```python
from build123d import *

# Parameters (mm, degrees)
SKETCH1_RX               = 240
SKETCH1_RY               = 110
BOSS_EXTRUDE1_DEPTH      = 200
SKETCH12_R               = 9
CUT_EXTRUDE8_DEPTH       = 332.209903234
CUT_EXTRUDE10_DEPTH      = 332.209903234
CUT_EXTRUDE10_DEPTH_BACK = 332.209903234
SKETCH15_W               = 200
SKETCH15_H               = 15


with BuildPart() as part:
    # Sketch1 → Boss-Extrude1 (new body)
    with BuildSketch(Plane.XY):
        with Locations((0, 0)):
            Ellipse(SKETCH1_RX, SKETCH1_RY)
    extrude(amount=-BOSS_EXTRUDE1_DEPTH)

    # Sketch12 → Cut-Extrude8 (cut, through all)
    with BuildSketch(Plane.XY):
        with Locations((175, -30)):
            Circle(SKETCH12_R)
        with Locations(Location((-175, -30, 0), (0, 0, 180))):
            Circle(SKETCH12_R)
    extrude(amount=-CUT_EXTRUDE8_DEPTH, mode=Mode.SUBTRACT)

    # Sketch15 → Cut-Extrude10 (cut, two sides: drawn at the far end of the back side and taken through both)
    with BuildSketch(Plane(origin=(0, 0, 0), x_dir=(0, 0, -1), z_dir=(1, 0, 0)).offset(-CUT_EXTRUDE10_DEPTH_BACK)):
        Polygon((0, 110), (0, 95), (200, -5), (200, 110), align=None)
        with Locations((100, -102.5)):
            Rectangle(SKETCH15_W, SKETCH15_H)
    extrude(amount=CUT_EXTRUDE10_DEPTH + CUT_EXTRUDE10_DEPTH_BACK, mode=Mode.SUBTRACT)


solid = part.part
```
Check sheet for the modelled part. Datum: model origin and axes. Units: mm. Coordinates: 2 decimals unless noted, no trailing zeros. Write each loop counter-clockwise with the first axis right and the second up, starting at its lowest first coordinate (ties: lowest second). Pieces come first, ordered by that corner, then holes. Notation, with made-up numbers: M -20.5,66 L 11.5,66 A14 cw 11.5,76 Z; hole C -37,20.5 d11. An arc over 180 degrees is marked long. Write item = value, one per line. Start each with the question number.
1. Go/stop test with flat-tipped pins: pin 1 (5 mm diameter, centred on x = 161.5, z = -102.5, fed in from -Y); pin 2 (8 mm diameter, centred on x = -10, z = -89.5, fed in from +Y); pin 3 (10 mm diameter, centred on x = 183, z = -169.5, fed in from +Y). Record where each tip stops, or that it passes through.
2. Sectioned sample at A-A (x = 29.5). Record the cut outline in (y, z), then the cut area to 3 significant figures.
3. Thickness scan on probe 1 along Y at (x, z) = (-175, -124.5); probe 2 along X at (y, z) = (-36.5, -29.5); probe 3 along Y at (x, z) = (-175, -127.5). Record the ranges inside material, lowest first.
4. Sectioned sample at B-B (y = -30). State how many separate pieces and enclosed holes the cut face has, then the cut area to 3 significant figures.
5. Mould release check, pull along X, two halves, no side actions. Record for faces 1 (the cylindrical face through (166, -30, -99)), 2 (the flat face through (-3, -49, -200)): pulls with the +X half, pulls with the -X half, needs draft (parallel to the pull), parting line crosses it, or undercut.
The answers:
q1.pin_1 = -82.4
q1.pin_2 = 52.25
q1.pin_3 = 12.75
q2.outline = M -95,-200 L -5,-200 L 95,0 L -95,0 Z
q2.area = 28,000 mm²
q3.probe_1 = -75.28 to -39, -21 to 32.75
q3.probe_2 = -226.4 to -181.22, -168.78 to 168.78, 181.22 to 226.4
q3.probe_3 = -75.28 to -39, -21 to 31.25
q4.separate_pieces = 3
q4.enclosed_holes = 0
q4.area = 85,200 mm²
q5.face_1 = undercut
q5.face_2 = needs draft
